Study the drawing (mm; zero at the part's minimum x, y, z) and answer. Give positions to 0.01 mm unless a question says otherwise; leave off trailing zeros. Order: outer loops, then holes, each group sorted by start corner. A loop starts at its lowest first (then second) coordinate and runs counter-clockwise, first axis right, second up. Notation, with made-up numbers: (15, 12.5) -> (42, 12.5) arc R25 ccw to (42, 39.5) -> close; hole circle Ø5 at (1, 58). An arc over 180 degrees is marked (long way). One line per question, with ' | ' between items. Start each with the question number.
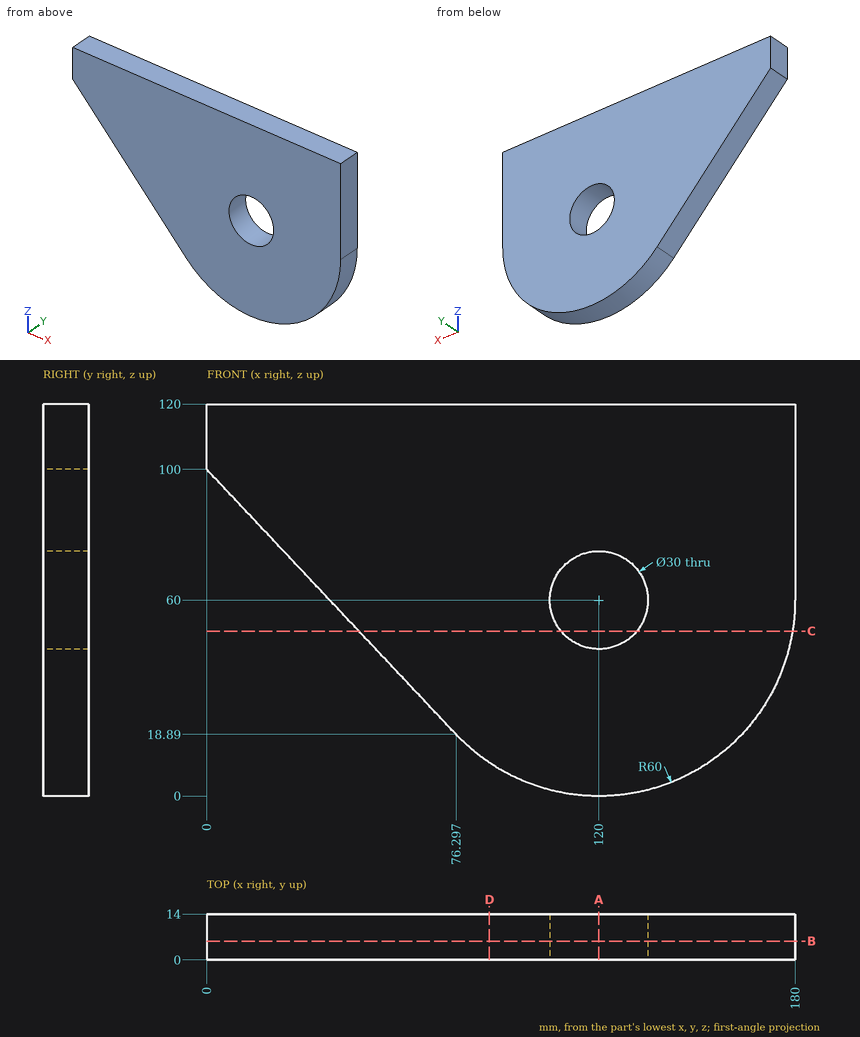
Q1. A cutting plane is placed at A-A, the plane x = 120. Determine the outline of the cut face in (y, z).
Q2. Find the intervals of material crossed by line 1 (Z direction, x = 120, y = 8.25); line 2 (X direction, y = 12.75, z = 48) (1 decimal); line 3 (X direction, y = 13.25, z = 50), in increasing order.
Q3. A cutting plane is placed at D-D, the plane x = 86.5. Determine the outline of the cut face in (y, z).
Q4. Given P1, Ø5, axis at x = 102, y = 3, coming from the -Z side; P2, Ø1, axis at x = 68.5, y = 6, coming from the -Z side; P3, Ø12, axis at x = 121.5, z = 98, coming from the -Y side; P4, Ø1.5, axis at y = 10, z = 75, coming from the -X side, each flat-ended and moving along its own axis, determine where each tip first touches the part or whether it passes through.
Q5. A cutting plane is placed at C-C, the plane z = 50.5. Determine the outline of the cut face in (x, y), then the cut area to 3 significant figures.
Q6. A cutting plane is placed at B-B, the plane y = 5.75. Determine the outline of the cut face in (x, z).
Geometry results:
1) outline: (0, 0) -> (14, 0) -> (14, 45) -> (0, 45) -> close; (0, 75) -> (14, 75) -> (14, 120) -> (0, 120) -> close
2) line 1: 0 to 45, 75 to 120 | line 2: 48.9 to 111, 129 to 178.8 | line 3: 47.03 to 108.82, 131.18 to 179.16
3) outline: (0, 10.22) -> (14, 10.22) -> (14, 120) -> (0, 120) -> close
4) P1: z = 2.04 | P2: z = 26.65 | P3: y = 0 | P4: x = 22.81
5) outline: (46.56, 0) -> (108.39, 0) -> (108.39, 14) -> (46.56, 14) -> close; (131.61, 0) -> (179.24, 0) -> (179.24, 14) -> (131.61, 14) -> close | area: 1,530 mm²
6) outline: (0, 100) -> (76.3, 18.89) arc R60 ccw to (180, 60) -> (180, 120) -> (0, 120) -> close; hole circle Ø30 at (120, 60)
